Autodesk Inventor part; units mm, degrees
ref_plane "YZ Plane" through (0, 0, 0) normal (1, 0, 0) x (0, 1, 0)
ref_plane "XZ Plane" through (0, 0, 0) normal (0, 1, 0) x (-1, 0, 0)
ref_plane "XY Plane" through (0, 0, 0) normal (0, 0, 1) x (1, 0, 0)
sketch "Sketch1" plane through (0, 0, 0) normal (0, 1, 0) x (-1, 0, 0)
  line L0 (10.1865, 69.048) -> (10.1865, -140.502)
  line L1 (10.1865, -140.502) -> (3.8365, -140.502)
  line L2 (3.8365, -140.502) -> (3.8365, -127.802)
  line L3 (3.8365, -127.802) -> (-2.5135, -127.802)
  line L4 (-2.5135, -127.802) -> (-2.5135, 56.348)
  line L5 (-2.5135, 56.348) -> (3.8365, 56.348)
  line L6 (3.8365, 56.348) -> (3.8365, 69.048)
  line L7 (3.8365, 69.048) -> (10.1865, 69.048)
  point P0 (0, 0)
  dimension "d0" = 184.15
  dimension "d1" = 6.35
  dimension "d2" = 6.35
  dimension "d3" = 12.7
  dimension "d4" = 12.7
  dimension "d5" = 6.35
extrude "Extrusion1" add sketch "Sketch1" along normal blind 127
sketch "Sketch2" plane through (-3.8365, 0, 69.048) normal (1, 0, 0) x (0, 0, -1)
  line L0 (12.7, 0) -> (0, 0)
  line L1 (0, 0) -> (0, 127)
  line L2 (0, 127) -> (12.7, 127)
  point P0 (69.048, 0)
  point P1 (6.35, 114.3)
  point P2 (6.35, 12.7)
  dimension "d8" = 12.7
  dimension "d9" = 6.35
  dimension "d10" = 6.35
  dimension "d11" = 12.7
hole "Hole1" at (-3.8365, 114.3, 62.698) at (-3.8365, 12.7, 62.698) direction (-1, 0, 0) diameter 4.0386 depth 25.4 tip angle 118
sketch "Sketch3" plane through (-3.8365, 0, -127.802) normal (1, 0, 0) x (0, 0, -1)
  line L0 (12.7, 0) -> (0, 0)
  line L1 (12.7, 0) -> (12.7, 127)
  line L2 (12.7, 127) -> (-196.85, 127)
  point P0 (-127.802, 0)
  point P1 (6.35, 114.3)
  point P2 (6.35, 12.7)
  dimension "d19" = 12.7
  dimension "d20" = 6.35
  dimension "d21" = 6.35
  dimension "d22" = 12.7
hole "Hole2" at (-3.8365, 114.3, -134.152) at (-3.8365, 12.7, -134.152) direction (-1, 0, 0) diameter 4.0386 depth 25.4 tip angle 118
sketch "Sketch4" plane through (-10.1865, 0, -140.502) normal (-1, 0, 0) x (0, 0, 1)
  line L0 (25.4, 120.65) -> (184.15, 120.65)
  line L1 (184.15, 120.65) -> (184.15, 6.35)
  line L2 (184.15, 6.35) -> (25.4, 6.35)
  line L3 (25.4, 6.35) -> (25.4, 120.65)
  line L4 (196.85, 127) -> (12.7, 127)
  line L5 (209.55, 0) -> (0, 0)
  line L6 (0, 0) -> (0, 127)
  line L7 (209.55, 0) -> (209.55, 127)
  point P0 (140.502, 0)
  dimension "d30" = 6.35
  dimension "d31" = 6.35
  dimension "d32" = 25.4
  dimension "d33" = 25.4
extrude "Extrusion2" cut sketch "Sketch4" against normal blind 3.175
sketch "Sketch5" plane through (0, 0, 0) normal (0, -1, 0) x (1, 0, 0)
  line L0 (2.5135, -127.802) -> (2.5135, 56.348)
  line L1 (-10.1865, -140.502) -> (-3.8365, -140.502)
  line L2 (-3.8365, 69.048) -> (-10.1865, 69.048)
  point P0 (0, 0)
  point P1 (-3.8365, -77.002)
  point P2 (-3.8365, 5.548)
  dimension "d36" = 6.35
  dimension "d37" = 6.35
  dimension "d38" = 63.5
  dimension "d39" = 63.5
hole "Hole3" at (-3.8365, 0, -77.002) at (-3.8365, 0, 5.548) direction (0, 1, 0) diameter 4.0386 depth 12.7 tip angle 118
properties part number "BatteryHighFront"
Read the model definition and answer for the solid it produces. Units are mm, in the model's axes. A direction names the side the tool comes from. Round coordinates to 2 decimals unless told otherwise and drop trailing zeros. Write each loop counter-clockwise with the first axis right and the second up, starting at its lowest first coordinate (ties: lowest second). Pieces come first, ordered by that corner, then holes.
Q1. Straight lines are drawn through the part: line 1 (Z direction, x = -8.5, y = 12.7); line 2 (Z direction, x = -5.25, y = 114.3); line 3 (Z direction, x = -9.5, y = 26). For each, find the intervals that lie inside material, in ascending order.
Values:
line 1: z = -140.5 to -136.17, -132.13 to -115.1, 43.65 to 60.68, 64.72 to 69.05
line 2: z = -140.5 to -136.17, -132.13 to 60.68, 64.72 to 69.05
line 3: z = -140.5 to -115.1, 43.65 to 69.05
Q2. Flat-ended cylindrical pins translate along their axes: P1, Ø1.9, axis at x = -2, y = 56, coming from the +Z side; P2, Ø4.5, axis at y = 12.7, z = -134.152, coming from the +X side; P3, Ø1.5, axis at x = -2, y = 111, coming from the -Z side. Find the tip coordinate at first contact, or state that the pin passes through.
Values:
P1: stops at z = 56.35
P2: stops at x = -3.84
P3: stops at z = -127.8
Q3. Find section B-B on z = -41. Determine the outline of the cut face in (x, y).
Values:
outline: (-10.19, 0) - (2.51, 0) - (2.51, 127) - (-10.19, 127) - (-10.19, 120.65) - (-7.01, 120.65) - (-7.01, 6.35) - (-10.19, 6.35) - close
Q4. Find section A-A on y = 114.3. Determine the outline of the cut face in (x, z), and give its area (3 significant figures).
Values:
outline: (-10.19, -140.5) - (-3.84, -140.5) - (-3.84, -136.17) - (-10.19, -136.17) - close; (-10.19, -132.13) - (-3.84, -132.13) - (-3.84, -127.8) - (2.51, -127.8) - (2.51, 56.35) - (-3.84, 56.35) - (-3.84, 60.68) - (-10.19, 60.68) - (-10.19, 43.65) - (-7.01, 43.65) - (-7.01, -115.1) - (-10.19, -115.1) - close; (-10.19, 64.72) - (-3.84, 64.72) - (-3.84, 69.05) - (-10.19, 69.05) - close
area: 1,940 mm2
Q5. A tool of negligible diameter and unlimited length cuts with its end or side. For faces 4 (the face through (-7.012, 64, -37)), 5 (the face through (-7.056, 12.093, 60.772)), 6 (the face through (-3.925, 6.439, -74.985)), 7 (the face through (-3.836, 63, -134)), 8 (the face through (-3.836, 63, 63)), from which of +Z, -Z, +X, -X, +Y, -Y can it reach the whole face along a straight path? Write none if from no direction.
Values:
face 4: -X
face 5: +X, -X
face 6: -Y
face 7: -Z, +X, +Y, -Y
face 8: +Z, +X, +Y, -Y
Q6. The mould has two halves that part along Y. Classify faces 1 (the face through (-1, 63, 56.348)), 2 (the face through (-4, 127, -34)), 3 (the face through (-7.06, 112.94, -132.66)): released by +Y, released by -Y, zero draft, split by the parting line, or undercut.
Values:
face 1: zero draft
face 2: released by +Y
face 3: undercut
